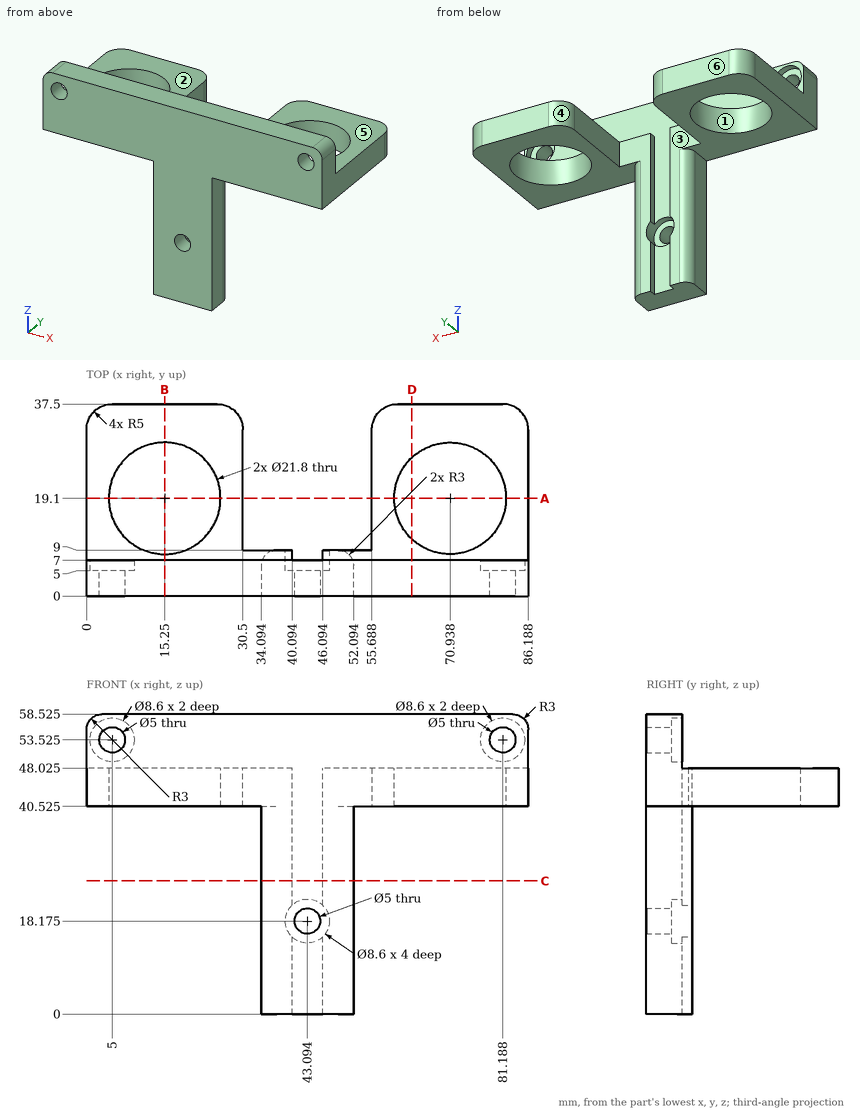
Drawing for the job (mm, zero at the part's lowest x, y, z). A direction names the side the tool comes from. Round coordinates to 2 decimals unless told otherwise and drop trailing zeros. Write each loop counter-clockwise with the first axis right and the second up, starting at its lowest first coordinate (ties: lowest second). Pieces come first, ordered by that corner, then holes. Notation, with made-up numbers: (9, 29) - (20, 29) arc R9 ccw to (20, 33) - close; hole circle Ø8 at (80, 63). An arc over 180 degrees is marked (long way). Use CSV: the item, a comma, the result in double quotes.
(1) Band-saw the part on A-A (y = 19.1). Give the number of separate pieces and of enclosed holes in the cut face, plus the area to 4 significant figures.
Response:
separate pieces,"4"
enclosed holes,"0"
area,"130.5 mm²"
(2) Band-saw the part on D-D (x = 63.5). Write the cut outline in (y, z) (1 decimal).
Response:
outline,"(0, 40.5) - (11.1, 40.5) - (11.1, 48) - (7, 48) - (7, 58.5) - (0, 58.5) - close; (27.1, 40.5) - (37.5, 40.5) - (37.5, 48) - (27.1, 48) - close"
(3) Pin check, flat tips, straight feed: P1, Ø1.8, axis at y = 2.5, z = 19, coming from the +X side; P2, Ø6.5, axis at x = 81.19, z = 53.52, coming from the +Y side; P3, Ø13, axis at x = 70.94, y = 19.1, coming from the +Z side; P4, Ø5, axis at x = 43.5, z = 7, coming from the +Y side. Stop position of each tip, or through.
Response:
P1,"x = 52.09"
P2,"y = 5"
P3,"through"
P4,"y = 7"
(4) 3-axis set-ups, long thin cutter, end or side, ignore diameter. For the marked faces 4, 5 and 6: which of +Z, -Z, +X, -X, +Y, -Y reach the whole face in a straight line?
Response:
face 4,"+Z, -Z, +Y"
face 5,"+Z, +X, -X, +Y"
face 6,"+Z, -Z, +X, -X, +Y"
(5) Band-saw the part on C-C (z = 26). Write the cut outline in (x, y).
Response:
outline,"(34.09, 0) - (52.09, 0) - (52.09, 6) arc R3 ccw to (49.09, 9) - (46.09, 9) - (46.09, 7) - (40.09, 7) - (40.09, 9) - (37.09, 9) arc R3 ccw to (34.09, 6) - close"
(6) Mould opens along Y. For the marked faces 1, 2 and 3 say: pulls with the +Y half, pulls with the -Y half, needs draft (parallel to the pull), parting line crosses it, or undercut.
Response:
face 1,"undercut"
face 2,"needs draft"
face 3,"pulls with the +Y half"
(7) Wall check: line 1 (X direction, y = 8, z = 43); line 2 (X direction, y = 18, z = 44.5); line 3 (Y direction, x = 36.5, z = 43). Give the ranges that are in metal, low to high.
Response:
line 1,"0 to 40.09, 46.09 to 86.19"
line 2,"0 to 4.41, 26.09 to 30.5, 55.69 to 60.09, 81.78 to 86.19"
line 3,"0 to 9"
(8) Band-saw the part on B-B (x = 15.25). Write the cut outline in (y, z) (3 decimals).
Response:
outline,"(0, 40.525) - (8.2, 40.525) - (8.2, 48.025) - (7, 48.025) - (7, 58.525) - (0, 58.525) - close; (30, 40.525) - (37.5, 40.525) - (37.5, 48.025) - (30, 48.025) - close"
